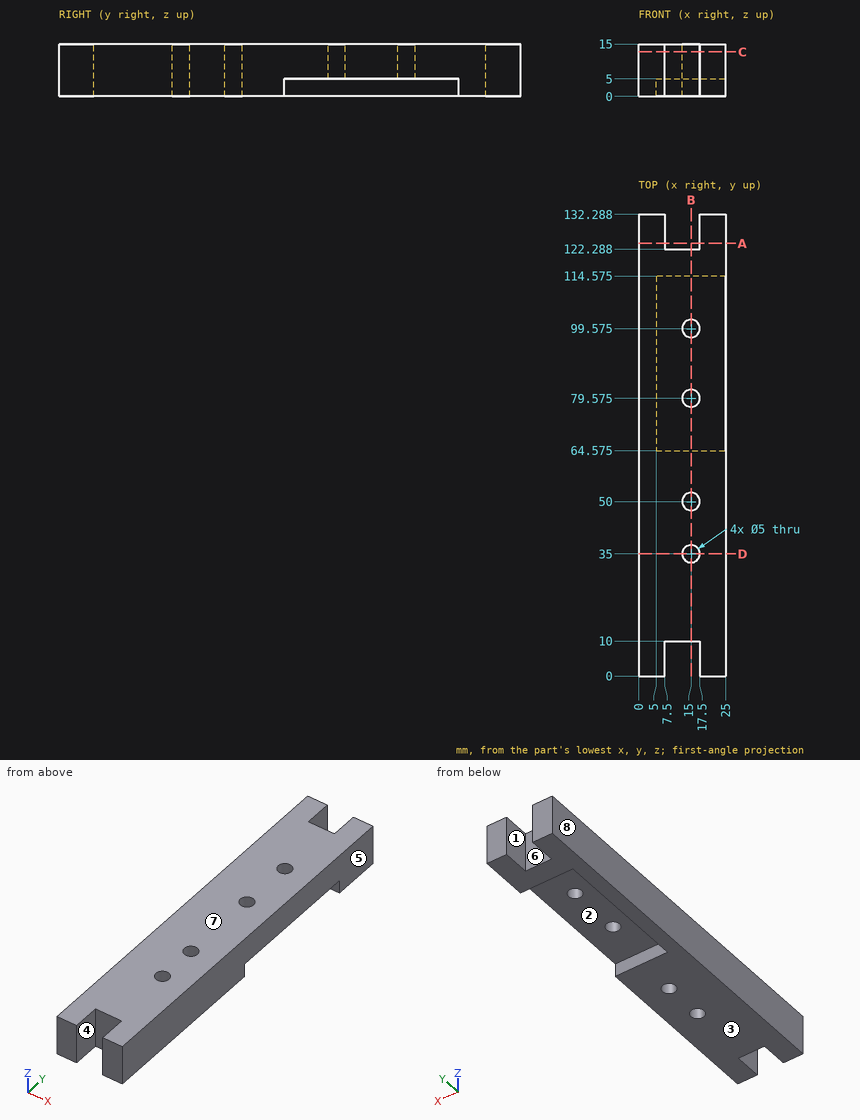
Geometry check sheet. Reference: drawing and pictorial views, mm from the part's lowest x, y, z. A direction names the side the tool comes from. Give positions to 0.01 mm unless a question says otherwise; leave off trailing zeros. Write each loop counter-clockwise with the first axis right and the second up, starting at its lowest first coordinate (ties: lowest second). Pieces come first, ordered by that corner, then holes. Notation, with made-up numbers: (57, 15.5) -> (77, 15.5) arc R37 cw to (77, 52.5) -> close; hole circle Ø6 at (9.5, 22). An arc over 180 degrees is marked (long way). One line per item, written item: value. Start each with the question number.
Item 1: Tool access check on the marked faces 1, 2, 3, 4 and 5. Record the directions out of +Z, -Z, +X, -X, +Y, -Y that give a thin tool (end or side, any length) a straight path to the whole face; none if there is none.
Item 2: Draft check along X on the marked faces 6, 7 and 8. Enter one of: +X half, -X half, draft (parallel to the pull), parting line (faces both ways), or undercut.
Item 3: Material ranges on probe 1 along Y at (x, z) = (15, 7) (1 decimal); probe 2 along X at (y, z) = (6.5, 12.75); probe 3 along Y at (x, z) = (6.25, 1.25) (1 decimal), recorded low to high. Write a range as from..to.
Item 4: Section check D-D on y = 35. Record the cut outline in (x, z), then the cut area to 3 significant figures.
Item 5: Section check B-B on x = 15. Record the cut outline in (y, z) (1 decimal), then the cut area to 3 significant figures.
Item 6: Section check C-C on z = 12.75. Record the cut outline in (x, y) (1 decimal), then the cut area to 3 significant figures.
Item 7: Gauge pin test, flat ends, axial feed: pin 1 (5 mm diameter, centred on x = 22, y = 101.5, fed in from -Z); pin 2 (1.5 mm diameter, centred on y = 77.5, z = 1.5, fed in from +X); pin 3 (3 mm diameter, centred on x = 13, z = 4.5, fed in from +Y). Record the tip position at first contact, or that the pin passes through.
Item 8: Section check A-A on y = 124. Record the cut outline in (x, z).
Results list:
1. face 1: +Z, -Z, +Y
1. face 2: -Z, +X
1. face 3: -Z, +X, -X, +Y, -Y
1. face 4: +Z, -Z, -Y
1. face 5: +Z, -Z, +X, +Y, -Y
2. face 6: undercut
2. face 7: draft
2. face 8: -X half
3. probe 1: 10..32.5, 37.5..47.5, 52.5..77.1, 82.1..97.1, 102.1..122.3
3. probe 2: 0..7.5, 17.5..25
3. probe 3: 0..64.6, 114.6..132.3
4. outline: (0, 0) -> (12.5, 0) -> (12.5, 15) -> (0, 15) -> close; (17.5, 0) -> (25, 0) -> (25, 15) -> (17.5, 15) -> close
4. area: 300 mm²
5. outline: (10, 0) -> (32.5, 0) -> (32.5, 15) -> (10, 15) -> close; (37.5, 0) -> (47.5, 0) -> (47.5, 15) -> (37.5, 15) -> close; (52.5, 0) -> (64.6, 0) -> (64.6, 5) -> (77.1, 5) -> (77.1, 15) -> (52.5, 15) -> close; (82.1, 5) -> (97.1, 5) -> (97.1, 15) -> (82.1, 15) -> close; (102.1, 5) -> (114.6, 5) -> (114.6, 0) -> (122.3, 0) -> (122.3, 15) -> (102.1, 15) -> close
5. area: 1,180 mm²
6. outline: (0, 0) -> (7.5, 0) -> (7.5, 10) -> (17.5, 10) -> (17.5, 0) -> (25, 0) -> (25, 132.3) -> (17.5, 132.3) -> (17.5, 122.3) -> (7.5, 122.3) -> (7.5, 132.3) -> (0, 132.3) -> close; hole circle Ø5 at (15, 35); hole circle Ø5 at (15, 50); hole circle Ø5 at (15, 79.6); hole circle Ø5 at (15, 99.6)
6. area: 3,030 mm²
7. pin 1: z = 5
7. pin 2: x = 5
7. pin 3: y = 122.29
8. outline: (0, 0) -> (7.5, 0) -> (7.5, 15) -> (0, 15) -> close; (17.5, 0) -> (25, 0) -> (25, 15) -> (17.5, 15) -> close
